The model under review builds one solid part; all positions refer to its coordinate system, in mm. Face numbers are marked on the shaded views. A direction names the side the tool comes from. Coordinates: 2 decimals unless noted, no trailing zeros. Write each loop counter-clockwise with the first axis right and the second up, starting at its lowest first coordinate (ties: lowest second). Pieces come first, ordered by that corner, then holes. Notation, with made-up numbers: (65.5, -16) - (77.5, -16) arc R21 ccw to (77.5, -9) - close; hole circle Ø7 at (81.5, 64). An arc over 180 degrees is marked (long way). Use one line per item in the form item = value. Start each with the question number.
```python
from build123d import *

# Parameters (mm, degrees)
SKETCH1_W                         = 9.8
SKETCH1_H                         = 11
BOSS_EXTRUDE1_BODY_DEPTH          = 2.2
FILLET1_BODYCORNERS_R             = 0.6
FILLET2_BODYFACES_R               = 0.4
CUT_EXTRUDE2_BASEINDENT_START     = -2.2
CUT_EXTRUDE2_BASEINDENT_DEPTH     = 0.1
BOSS_EXTRUDE4_BASESTUDS_START     = -2.1
SKETCH5_R                         = 0.75
SKETCH5_R_2                       = 0.45
SKETCH5_R_3                       = 0.4
BOSS_EXTRUDE4_BASESTUDS_DEPTH     = 0.8
BOSS_EXTRUDE5_PINS_DEPTH          = 2.2
BOSS_EXTRUDE5_PINS_DEPTH_BACK     = 4.8
BOSS_EXTRUDE5_PINS_START          = -2.1
SKETCH6_W                         = 1
SKETCH6_H                         = 0.2
CHAMFER2_PINS_SIZE                = 0.4
BOSS_EXTRUDE6_KNOBEDGE_START      = -2.2
SKETCH7_R                         = 2.6
SKETCH7_R_2                       = 2
BOSS_EXTRUDE6_KNOBEDGE_DEPTH      = 4.5
CUT_EXTRUDE3_SHAFTHOLE_DEPTH      = 17.26806688
CUT_EXTRUDE3_SHAFTHOLE_DEPTH_BACK = 15.16806688
CUT_EXTRUDE3_SHAFTHOLE_START      = -2.1
SKETCH8_R                         = 2
CUT_EXTRUDE4_DETAIL_START         = 2.2
SKETCH9_R                         = 0.35
CUT_EXTRUDE4_DETAIL_DEPTH         = 0.1


with BuildPart() as part:
    # Sketch1 → Boss-Extrude1_Body (new, symmetric)
    with BuildSketch(Plane.XY):
        with Locations((-4.9, -5.5)):
            Rectangle(SKETCH1_W, SKETCH1_H)
    extrude(amount=BOSS_EXTRUDE1_BODY_DEPTH, both=True)

    # Fillet1_BodyCorners
    fillet1_bodycorners_edges = [part.edges().sort_by_distance(p)[0] for p in [
        (0, -11, 0),
        (-9.8, -11, 0),
        (-9.8, 0, 0),
        (0, 0, 0),
    ]]
    fillet(fillet1_bodycorners_edges, radius=FILLET1_BODYCORNERS_R)

    # Fillet2_BodyFaces
    fillet2_bodyfaces_edges = [part.edges().sort_by_distance(p)[0] for p in [
        (-9.8, -5.5, -2.2),
        (-9.8, -5.5, 2.2),
        (0, -5.5, -2.2),
        (-4.9, -11, -2.2),
        (-4.9, 0, -2.2),
        (-0.175735931, -0.175735931, -2.2),
        (-0.175735931, -10.824264069, -2.2),
        (-9.624264069, -10.824264069, -2.2),
        (-9.624264069, -0.175735931, -2.2),
        (-4.9, 0, 2.2),
        (0, -5.5, 2.2),
        (-4.9, -11, 2.2),
        (-0.175735931, -0.175735931, 2.2),
        (-0.175735931, -10.824264069, 2.2),
        (-9.624264069, -10.824264069, 2.2),
        (-9.624264069, -0.175735931, 2.2),
    ]]
    fillet(fillet2_bodyfaces_edges, radius=FILLET2_BODYFACES_R)

    # Sketch4 → Cut-Extrude2_BaseIndent (cut)
    with BuildSketch(Plane.XY.offset(CUT_EXTRUDE2_BASEINDENT_START)):
        with BuildLine():
            Line((-0.6, -0.4), (-9.2, -0.4))
            ThreePointArc((-9.2, -0.4), (-9.341421356, -0.458578644), (-9.4, -0.6))
            Line((-9.4, -0.6), (-9.4, -10.4))
            ThreePointArc((-9.4, -10.4), (-9.341421356, -10.541421356), (-9.2, -10.6))
            Line((-9.2, -10.6), (-0.6, -10.6))
            ThreePointArc((-0.6, -10.6), (-0.458578644, -10.541421356), (-0.4, -10.4))
            Line((-0.4, -10.4), (-0.4, -0.6))
            ThreePointArc((-0.4, -0.6), (-0.458578644, -0.458578644), (-0.6, -0.4))
        make_face()
    extrude(amount=CUT_EXTRUDE2_BASEINDENT_DEPTH, mode=Mode.SUBTRACT)

    # Sketch5 → Boss-Extrude4_BaseStuds (add)
    # profile 1 of 3: a face of its own
    with BuildSketch(Plane.XY.offset(BOSS_EXTRUDE4_BASESTUDS_START)):
        with Locations(Location((-4.9, -1.1, 0), (0, 0, 68.960530219))):
            Circle(SKETCH5_R)
        with Locations(Location((-4.9, -1.1, 0), (0, 0, 180))):
            Circle(SKETCH5_R_2, mode=Mode.SUBTRACT)
    # profile 2 of 3: a face of its own
    with BuildSketch(Plane.XY.offset(BOSS_EXTRUDE4_BASESTUDS_START)):
        with Locations(Location((-1.35, -9.7, 0), (0, 0, 180))):
            Circle(SKETCH5_R_3)
    # profile 3 of 3: a face of its own
    with BuildSketch(Plane.XY.offset(BOSS_EXTRUDE4_BASESTUDS_START)):
        with Locations(Location((-8.45, -9.7, 0), (0, 0, 180))):
            Circle(SKETCH5_R_3)
    extrude(amount=-BOSS_EXTRUDE4_BASESTUDS_DEPTH)

    # Sketch6 → Boss-Extrude5_Pins (add, two sides: drawn at the far end of the back side and taken through both)
    with BuildSketch(Plane.XY.offset(BOSS_EXTRUDE5_PINS_START - BOSS_EXTRUDE5_PINS_DEPTH_BACK)):
        with Locations((-2.5, -0.11)):
            Rectangle(SKETCH6_W, SKETCH6_H)
        with Locations((-7.3, -0.11)):
            Rectangle(SKETCH6_W, SKETCH6_H)
        with Locations((-4.9, -10.89)):
            Rectangle(SKETCH6_W, SKETCH6_H)
    extrude(amount=BOSS_EXTRUDE5_PINS_DEPTH + BOSS_EXTRUDE5_PINS_DEPTH_BACK)

    # Chamfer2_Pins
    chamfer2_pins_edges = [part.edges().sort_by_distance(p)[0] for p in [
        (-2, -0.11, -6.9),
        (-3, -0.11, -6.9),
        (-6.8, -0.11, -6.9),
        (-7.8, -0.11, -6.9),
        (-4.4, -10.89, -6.9),
        (-5.4, -10.89, -6.9),
    ]]
    chamfer(chamfer2_pins_edges, length=CHAMFER2_PINS_SIZE)

    # Sketch7 → Boss-Extrude6_KnobEdge (add)
    with BuildSketch(Plane.XY.offset(BOSS_EXTRUDE6_KNOBEDGE_START)):
        with Locations(Location((-4.9, -6.2, 0), (0, 0, 180))):
            Circle(SKETCH7_R)
        with Locations(Location((-4.9, -6.2, 0), (0, 0, 180))):
            Circle(SKETCH7_R_2, mode=Mode.SUBTRACT)
    extrude(amount=BOSS_EXTRUDE6_KNOBEDGE_DEPTH)

    # Sketch8 → Cut-Extrude3_ShaftHole (cut, two sides: drawn at the far end of the back side and taken through both)
    with BuildSketch(Plane.XY.offset(CUT_EXTRUDE3_SHAFTHOLE_START - CUT_EXTRUDE3_SHAFTHOLE_DEPTH_BACK)):
        with Locations(Location((-4.9, -6.2, 0), (0, 0, 180))):
            Circle(SKETCH8_R)
    extrude(amount=CUT_EXTRUDE3_SHAFTHOLE_DEPTH + CUT_EXTRUDE3_SHAFTHOLE_DEPTH_BACK, mode=Mode.SUBTRACT)

    # Sketch9 → Cut-Extrude4_Detail (cut)
    with BuildSketch(Plane.XY.offset(CUT_EXTRUDE4_DETAIL_START)):
        with Locations(Location((-7.725, -4.2, 0), (0, 0, 180))):
            Circle(SKETCH9_R)
        with Locations(Location((-2.075, -4.2, 0), (0, 0, 180))):
            Circle(SKETCH9_R)
        with Locations(Location((-4.9, -9.4, 0), (0, 0, 180))):
            Circle(SKETCH9_R)
    extrude(amount=-CUT_EXTRUDE4_DETAIL_DEPTH, mode=Mode.SUBTRACT)


solid = part.part
```
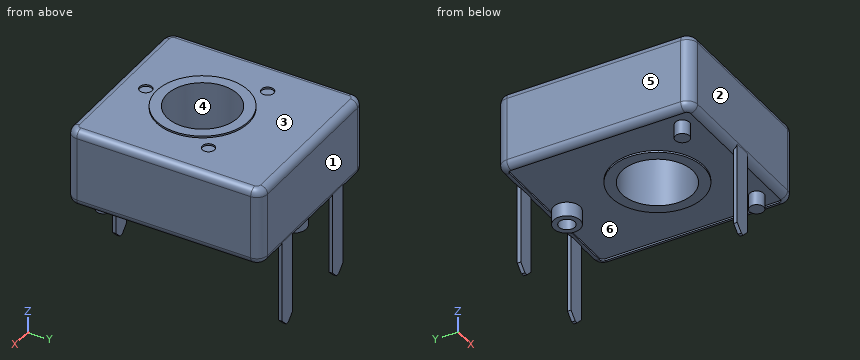
1. Take a section at C-C (y = -1.1). State the section outline as (x, z) points, plus the area to 3 significant figures.
2. Take a section at A-A (z = -5). State the section outline as (x, y) points.
3. For P1, Ø0.8, axis at x = -5, z = -5, coming from the +Y side; P2, Ø2.5, axis at x = -7, y = -6.5, coming from the -Z side; P3, Ø0.8, axis at x = -7.5, y = -4, coming from the +Z side, all flat-tipped, find the tip position at first contact; note any pin that passes through.
4. For L1, parallel to Y at x = -4.9, z = 2.25; L2, parallel to X at y = -6.2, z = -1; L3, parallel to Z at x = -9, y = -6.25, list the stretches that pass through material, from the lowest coordinate up.
5. The part is to be moulded in two halves that separate along Y. For the marked faces 1, 2, 3 and 4, say which applies: released by +Y, released by -Y, zero draft, split by the parting line, or undercut.
6. For the marked faces 5 and 6, list the 3-axis set-ups (+Z, -Z, +X, -X, +Y, -Y) from which the entire face can be reached by the end or side of a thin tool; tool diameter is ignored.
7. Take a section at B-B (x = -6). State the section outline as (y, z) points, plus the area to 3 significant figures.
8. Take a section at D-D (z = -1.5). State the section outline as (x, y) points.
Returned:
q1.outline = (-9.8, -1.8) arc R0.4 ccw to (-9.4, -2.2) - (-9.4, -2.1) - (-5.65, -2.1) - (-5.65, -2.9) - (-5.35, -2.9) - (-5.35, -2.1) - (-4.45, -2.1) - (-4.45, -2.9) - (-4.15, -2.9) - (-4.15, -2.1) - (-0.4, -2.1) - (-0.4, -2.2) arc R0.4 ccw to (0, -1.8) - (0, 1.8) arc R0.4 ccw to (-0.4, 2.2) - (-9.4, 2.2) arc R0.4 ccw to (-9.8, 1.8) - close
q1.area = 42.6 mm²
q2.outline = (-7.8, -0.21) - (-6.8, -0.21) - (-6.8, -0.01) - (-7.8, -0.01) - close; (-5.4, -10.99) - (-4.4, -10.99) - (-4.4, -10.79) - (-5.4, -10.79) - close; (-3, -0.21) - (-2, -0.21) - (-2, -0.01) - (-3, -0.01) - close
q3.P1 = -10.79
q3.P2 = -2.2
q3.P3 = 2.2
q4.L1 = -8.8 to -8.2, -4.2 to -3.6
q4.L2 = -9.8 to -6.9, -2.9 to 0
q4.L3 = -2.1 to 2.2
q5.face_1 = released by +Y
q5.face_2 = released by -Y
q5.face_3 = zero draft
q5.face_4 = undercut
q6.face_5 = +Z, -Z, -X, +Y, -Y
q6.face_6 = -Z
q7.outline = (-11, -1.8) arc R0.4 ccw to (-10.6, -2.2) - (-10.6, -2.1) - (-8.56, -2.1) - (-8.56, -2.2) - (-7.87, -2.2) - (-7.87, 2.3) - (-8.56, 2.3) - (-8.56, 2.2) - (-10.6, 2.2) arc R0.4 ccw to (-11, 1.8) - close; (-4.53, -2.2) - (-3.84, -2.2) - (-3.84, -2.1) - (-0.4, -2.1) - (-0.4, -2.2) arc R0.4 ccw to (0, -1.8) - (0, 1.8) arc R0.4 ccw to (-0.4, 2.2) - (-3.84, 2.2) - (-3.84, 2.3) - (-4.53, 2.3) - close
q7.area = 33.2 mm²
q8.outline = (-9.8, -10.4) arc R0.6 ccw to (-9.2, -11) - (-0.6, -11) arc R0.6 ccw to (0, -10.4) - (0, -0.6) arc R0.6 ccw to (-0.6, 0) - (-9.2, 0) arc R0.6 ccw to (-9.8, -0.6) - close; hole circle Ø4 at (-4.9, -6.2)
